from build123d import *

# Parameters (mm, degrees)
SKETCH1_R           = 49.5046
BOSS_EXTRUDE1_DEPTH = 5.08
SKETCH2_R           = 47.625
BOSS_EXTRUDE2_DEPTH = 5.08
SKETCH3_R           = 11.176
SKETCH3_R_2         = 3.96875
SKETCH3_R_3         = 9.525
CUT_EXTRUDE1_DEPTH  = 11.16
SKETCH7_R           = 65.421404769
CUT_EXTRUDE3_DEPTH  = 5.08


with BuildPart() as part:
    # Sketch1 → Boss-Extrude1 (new body)
    with BuildSketch(Plane.XY):
        Circle(SKETCH1_R)
    extrude(amount=BOSS_EXTRUDE1_DEPTH)

    # Sketch2 → Boss-Extrude2 (add)
    with BuildSketch(Plane.XY.offset(5.08)):
        Circle(SKETCH2_R)
    extrude(amount=BOSS_EXTRUDE2_DEPTH)

    # Sketch3 → Cut-Extrude1 (cut, through all)
    with BuildSketch(Plane.XY.offset(10.16)):
        with Locations((-12.7, -31.166793627)):
            Circle(SKETCH3_R)
        with Locations((12.7, -31.166793627)):
            Circle(SKETCH3_R)
        with Locations((-36.83, 0)):
            Circle(SKETCH3_R_2)
        with Locations((36.83, 0)):
            Circle(SKETCH3_R_2)
        Circle(SKETCH3_R_3)
    extrude(amount=-CUT_EXTRUDE1_DEPTH, mode=Mode.SUBTRACT)

    # Sketch7 → Cut-Extrude3 (cut)
    with BuildSketch(Plane(origin=(0, 0, 0), x_dir=(-1, 0, 0), z_dir=(0, 0, -1))):
        Circle(SKETCH7_R)
    extrude(amount=-CUT_EXTRUDE3_DEPTH, mode=Mode.SUBTRACT)


solid = part.part
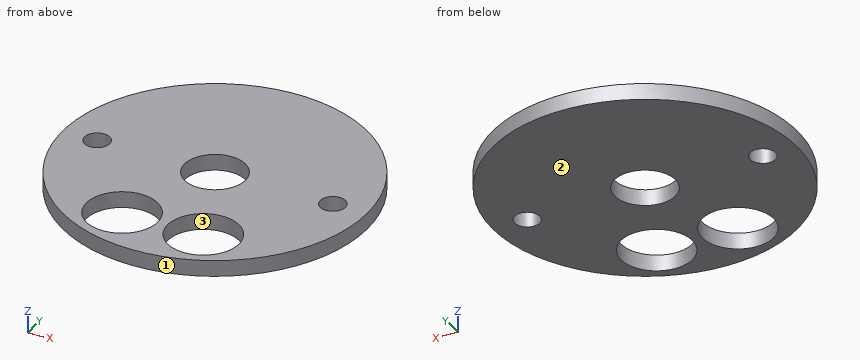
For this review, take the finished solid that the model builds, in its own axes (mm). Face numbers are marked on the shaded views. Give positions to 0.01 mm unless a question says otherwise; leave off trailing zeros. Loops run counter-clockwise (first coordinate to the right, second up) from the corner with the lowest first, then second, coordinate; pieces in that order, holes last. Notation, with made-up numbers: M 27,86.5 L 83,86.5 A13 cw 83,94.5 Z; hole C 25.5,32 d2. An arc over 180 degrees is marked long. Put each result on its own line as item: value. Start each with the question number.
(1) Wall thickness on L1, parallel to X at y = -1, z = 7.4; L2, parallel to X at y = -27, z = 6.05; L3, parallel to Y at x = 17.5, z = 7.5: over which ranges is each line inside the solid? List them lowest first.
(2) Add section B-B, the plane y = 0. Write out the cut boundary in (x, z) (3 decimals).
(3) The part is to be moulded in two halves that separate along X. For the marked faces 1, 2 and 3, say which applies: +X half, -X half, draft (parallel to the pull), parting line (faces both ways), or undercut.
(4) For pin 1 (3 mm diameter, centred on x = -11, z = 6.5, fed in from -Y); pin 2 (13.5 mm diameter, centred on x = 12.7, y = -31.17, fed in from +Z); pin 3 (1.5 mm diameter, centred on x = -1, z = 9.5, fed in from -Y); pin 4 (1 mm diameter, centred on x = 23.5, z = 9, fed in from -Y), all flat-tipped, find the tip position at first contact; note any pin that passes through.
(5) Add section C-C, the plane y = -23. Write out the cut boundary in (x, z).
(6) Add section A-A, the plane x = 0. Write out the cut boundary in (y, z) (3 decimals).
(7) Add section D-D, the plane z = 7.45. Give the number of separate pieces and of enclosed holes in the cut face, then the cut area to 3 significant figures.
Result:
1. L1: x = -47.61 to -40.67, -32.99 to -9.47, 9.47 to 32.99, 40.67 to 47.61
1. L2: x = -39.23 to -23.07, -2.33 to 2.33, 23.07 to 39.23
1. L3: y = -44.29 to -41.26, -21.07 to 44.29
2. outline: M -47.625,5.08 L -40.799,5.08 L -40.799,10.16 L -47.625,10.16 Z; M -32.861,5.08 L -9.525,5.08 L -9.525,10.16 L -32.861,10.16 Z; M 9.525,5.08 L 32.861,5.08 L 32.861,10.16 L 9.525,10.16 Z; M 40.799,5.08 L 47.625,5.08 L 47.625,10.16 L 40.799,10.16 Z
3. face 1: parting line
3. face 2: draft
3. face 3: undercut
4. pin 1: stops at y = -46.67
4. pin 2: passes through
4. pin 3: stops at y = -47.62
4. pin 4: stops at y = -41.7
5. outline: M -41.7,5.08 L -20.33,5.08 L -20.33,10.16 L -41.7,10.16 Z; M -5.07,5.08 L 5.07,5.08 L 5.07,10.16 L -5.07,10.16 Z; M 20.33,5.08 L 41.7,5.08 L 41.7,10.16 L 20.33,10.16 Z
6. outline: M -47.625,5.08 L -9.525,5.08 L -9.525,10.16 L -47.625,10.16 Z; M 9.525,5.08 L 47.625,5.08 L 47.625,10.16 L 9.525,10.16 Z
7. separate pieces: 1
7. enclosed holes: 5
7. area: 5,960 mm^2
